from build123d import *

# Parameters (mm, degrees)
BOSS_EXTRUDE1_DEPTH = 40
CUT_EXTRUDE1_DEPTH  = 30


with BuildPart() as part:
    # Sketch1 → Boss-Extrude1 (new body)
    with BuildSketch(Plane.XY):
        Polygon((0, 0), (10, 0), (0, 5), align=None)
    extrude(amount=BOSS_EXTRUDE1_DEPTH)

    # Sketch3 → Cut-Extrude1 (cut)
    with BuildSketch(Plane.ZY):
        Polygon((5, 5), (0, 1.537620853), (0, 5), align=None)
        Polygon((35, 5), (40, 5), (40, 1.537620853), align=None)
    extrude(amount=-CUT_EXTRUDE1_DEPTH, mode=Mode.SUBTRACT)


solid = part.part
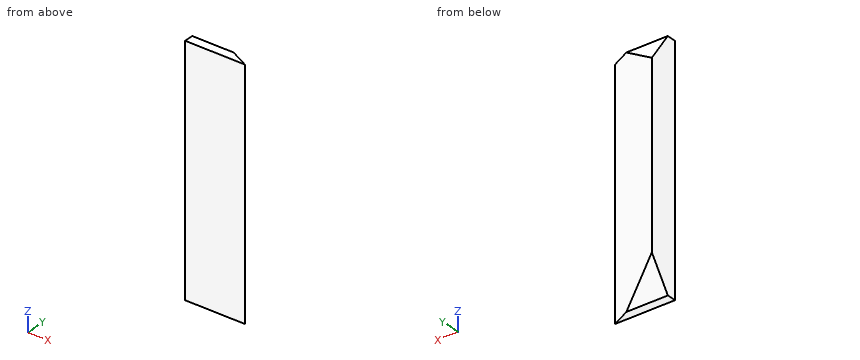
Geometry check sheet. Reference: the model listing, model coordinates, mm. Round coordinates to 2 decimals unless told otherwise and drop trailing zeros. Loops run counter-clockwise (first coordinate to the right, second up) from the corner with the lowest first, then second, coordinate; pieces in that order, holes last. Notation, with made-up numbers: (41.5, -27) - (50.5, -27) arc R11 ccw to (50.5, -8) - close; hole circle Ø9 at (88, 48). An arc over 180 degrees is marked (long way). Answer as CSV lines item,"result".
(1) Cross-section at C-C, the plane y = 1.05. Enter the section's corners in (x, z), and give its area (3 significant figures).
Output values:
outline,"(0, 0) - (7.9, 0) - (7.9, 40) - (0, 40) - close"
area,"316 mm²"
(2) Depth check by flat-ended pin: pin 1 Ø2 at (x, y) = (6, 3) entering from -Z. Enter the tip coordinate at first touch or a pass-through.
Output values:
pin 1,"stops at z = 0.67"
(3) Cross-section at B-B, the plane z = 34. Enter the section's corners in (x, y).
Output values:
outline,"(0, 0) - (10, 0) - (0, 5) - close"
(4) Cross-section at A-A, the plane x = 8.5. Enter the section's corners in (y, z), and give its area (3 significant figures).
Output values:
outline,"(0, 0) - (0.75, 0) - (0.75, 40) - (0, 40) - close"
area,"30.0 mm²"
(5) Cross-section at D-D, the plane x = 0.5. Enter the section's corners in (y, z).
Output values:
outline,"(0, 0) - (1.54, 0) - (4.75, 4.64) - (4.75, 35.36) - (1.54, 40) - (0, 40) - close"
(6) Material ranges on line 1 along X through (y, z) = (2.5, 18); line 2 along X through (y, z) = (0.75, 17); line 3 along Y through (x, z) = (1.25, 27) (3 decimals), recorded low to high.
Output values:
line 1,"x = 0 to 5"
line 2,"x = 0 to 8.5"
line 3,"y = 0 to 4.375"
